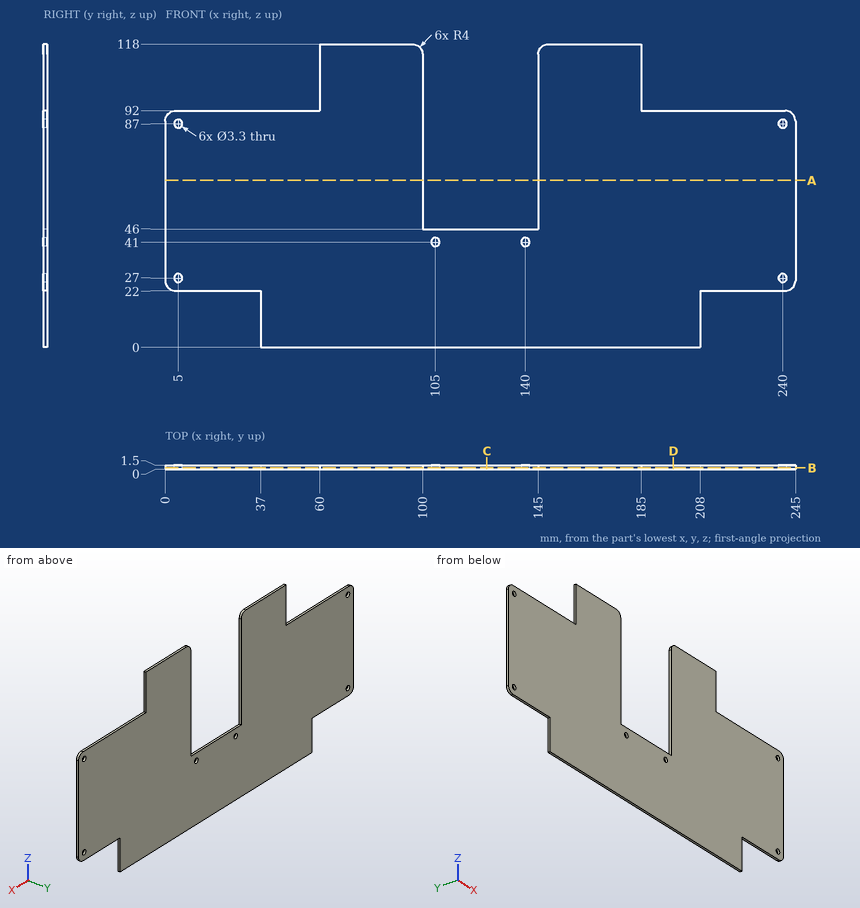
Geometry: see drawing. Coordinates: mm, zero at the bounding-box minimum. Coordinates: 2 decimals unless noted, no trailing zeros. Loops run counter-clockwise (first coordinate to the right, second up) from the corner with the lowest first, then second, coordinate; pieces in that order, holes last. Notation, with made-up numbers: (89.25, -16) - (141.25, -16) arc R21 ccw to (141.25, 18) - close; hole circle Ø3 at (65, -37.75). An arc over 180 degrees is marked (long way). Put each result on its own line as item: value. Start each with the question number.
Q1. Pin query (flat end, axial travel): pin 1 Ø2.5 at (x, z) = (5, 87) entering from +Y; pin 2 Ø0.8 at (x, y) = (228.5, 1) entering from -Z; pin 3 Ø0.8 at (y, z) = (1, 12.5) entering from -X. Return the tip coordinate at first contact, or that it passes through.
Q2. Cut plane A-A, the plane z = 65. Return loops of the section in (x, y).
Q3. Cut plane D-D, the plane x = 197.5. Return loops of the section in (y, z), and give its area (3 significant figures).
Q4. Cut plane B-B, the plane y = 0.55. Return loops of the section in (x, z).
Q5. Cut plane C-C, the plane x = 125. Return loops of the section in (y, z), and give its area (3 significant figures).
Q6. Line query: line 1 (Z direction, x = 240, y = 1.05); line 2 (X direction, y = 1.1, z = 27); line 3 (X direction, y = 0.5, z = 87). Output: solid intervals per line, ascending.
Filled sheet:
1. pin 1: through
1. pin 2: z = 22
1. pin 3: x = 37
2. outline: (0, 0) - (100, 0) - (100, 1.5) - (0, 1.5) - close; (145, 0) - (245, 0) - (245, 1.5) - (145, 1.5) - close
3. outline: (0, 0) - (1.5, 0) - (1.5, 92) - (0, 92) - close
3. area: 138 mm²
4. outline: (0, 26) arc R4 ccw to (4, 22) - (37, 22) - (37, 0) - (208, 0) - (208, 22) - (241, 22) arc R4 ccw to (245, 26) - (245, 88) arc R4 ccw to (241, 92) - (185, 92) - (185, 118) - (149, 118) arc R4 ccw to (145, 114) - (145, 46) - (100, 46) - (100, 114) arc R4 ccw to (96, 118) - (60, 118) - (60, 92) - (4, 92) arc R4 ccw to (0, 88) - close; hole circle Ø3.3 at (5, 27); hole circle Ø3.3 at (5, 87); hole circle Ø3.3 at (105, 41); hole circle Ø3.3 at (140, 41); hole circle Ø3.3 at (240, 27); hole circle Ø3.3 at (240, 87)
5. outline: (0, 0) - (1.5, 0) - (1.5, 46) - (0, 46) - close
5. area: 69.0 mm²
6. line 1: 22 to 25.35, 28.65 to 85.35, 88.65 to 92
6. line 2: 0 to 3.35, 6.65 to 238.35, 241.65 to 245
6. line 3: 0 to 3.35, 6.65 to 100, 145 to 238.35, 241.65 to 245
